CAD build for the part. Positions are in the model's coordinates, mm. Coordinates: 2 decimals unless noted, no trailing zeros. Order: outer loops, then holes, each group sorted by start corner. A loop starts at its lowest first (then second) coordinate and runs counter-clockwise, first axis right, second up. Notation, with made-up numbers: M 12.25,69.5 L 56.25,69.5 A20 cw 56.25,79.5 Z; hole C 7.25,53.25 d10. An arc over 180 degrees is marked long. One line per item, written item: value.
from build123d import *

# Parameters (mm, degrees)
F0_R     = 1.5
F0_R_2   = 1
F1_DEPTH = 1.6


with BuildPart() as f1:
    # F0 (on Front) → F1 (new body)
    with BuildSketch(Plane.XZ):
        with BuildLine():
            Line((35.5, 50), (-35.5, 50))
            Line((-35.5, 50), (-35.5, 35))
            Line((-35.5, 35), (-35.5, -27))
            Line((-35.5, -27), (-35.5, -50))
            Line((-35.5, -50), (35.5, -50))
            Line((35.5, -50), (35.5, -12.5))
            Line((35.5, -12.5), (45.5, -12.5))
            ThreePointArc((45.5, -12.5), (46.9142135624, -11.9142135624), (47.5, -10.5))
            Line((47.5, -10.5), (47.5, 10.5))
            ThreePointArc((47.5, 10.5), (46.9142135624, 11.9142135624), (45.5, 12.5))
            Line((45.5, 12.5), (35.5, 12.5))
            Line((35.5, 12.5), (35.5, 50))
        make_face()
        with Locations((-31, -45.5)):
            Circle(F0_R, mode=Mode.SUBTRACT)
        with Locations((-15, -9.5)):
            Circle(F0_R_2, mode=Mode.SUBTRACT)
        with Locations((-10, -9.5)):
            Circle(F0_R_2, mode=Mode.SUBTRACT)
        with Locations((-12.5, -3.5)):
            Circle(F0_R, mode=Mode.SUBTRACT)
        with Locations((31, -45.5)):
            Circle(F0_R, mode=Mode.SUBTRACT)
        with BuildLine():
            ThreePointArc((-12.5, 7.5), (-10.9878693139, 6.99084424), (-10.0916666667, 5.6707686304))
            ThreePointArc((-10.0916666667, 5.6707686304), (-8.9906023558, 5.9331845119), (-8.35, 5))
            ThreePointArc((-8.35, 5), (-8.9906023558, 4.0668154881), (-10.0916666667, 4.3292313696))
            ThreePointArc((-10.0916666667, 4.3292313696), (-12.5, 2.5), (-14.9083333333, 4.3292313696))
            ThreePointArc((-14.9083333333, 4.3292313696), (-16.65, 5), (-14.9083333333, 5.6707686304))
            ThreePointArc((-14.9083333333, 5.6707686304), (-14.0121306861, 6.99084424), (-12.5, 7.5))
        make_face(mode=Mode.SUBTRACT)
        with Locations((-31, 45.5)):
            Circle(F0_R, mode=Mode.SUBTRACT)
        with Locations((31, 45.5)):
            Circle(F0_R, mode=Mode.SUBTRACT)
    extrude(amount=-F1_DEPTH)


solid = f1.part
Q1. Slice it at A-A (z = 45.5). List the corners of the cut face in (x, y).
Recorded:
outline: M -35.5,0 L -32.5,0 L -32.5,1.6 L -35.5,1.6 Z; M -29.5,0 L 29.5,0 L 29.5,1.6 L -29.5,1.6 Z; M 32.5,0 L 35.5,0 L 35.5,1.6 L 32.5,1.6 Z
Q2. Pin check, flat tips, straight feed: pin 1 Ø2.5 at (x, z) = (-31, -45.5) entering from +Y; pin 2 Ø0.5 at (x, y) = (41.5, 1) entering from -Z; pin 3 Ø0.5 at (y, z) = (1, -28.5) entering from +X. Stop position of each tip, or through.
Recorded:
pin 1: passes through
pin 2: stops at z = -12.5
pin 3: stops at x = 35.5
Q3. Slice it at B-B (y = 0.5). Give the number of separate pieces and of enclosed holes in the cut face, plus the area to 3 significant figures.
Recorded:
separate pieces: 1
enclosed holes: 8
area: 7,330 mm^2
Q4. Slice it at C-C (z = 22). List the corners of the cut face in (x, y).
Recorded:
outline: M -35.5,0 L 35.5,0 L 35.5,1.6 L -35.5,1.6 Z
Q5. Mould opens along X. For faces 1 (the face through (5, 1.6, 1)), 2 (the face through (-14.046, 0.789, -9.2)), 3 (the face through (46.9, 0.79, -11.93)) say: released by +X, released by -X, zero draft, split by the parting line, or undercut.
Recorded:
face 1: zero draft
face 2: undercut
face 3: released by +X
Q6. Drill centre lines: line 1 along Z through (x, y) = (-31, 0.9); line 2 along Z through (x, y) = (-10, 0.55); line 3 along X through (y, z) = (1.25, -32.5). Where is each one in solid material? Low to high.
Recorded:
line 1: z = -50 to -47, -44 to 44, 47 to 50
line 2: z = -50 to -10.5, -8.5 to 4.24, 5.76 to 50
line 3: x = -35.5 to 35.5
